Input: part model. Units: mm. Frame: model coordinates. Face numbers are marked on the shaded views. A direction names the side the tool comes from. Round coordinates to 2 decimals unless told otherwise and drop trailing zeros. Write each loop counter-clockwise with the first axis right and the second up, starting at its lowest first coordinate (ties: lowest second). Pieces come first, ordered by that corner, then holes. Notation, with made-up numbers: (61, 36.25) - (87, 36.25) arc R22 cw to (87, 74.25) - close; hole circle Ø5 at (78.25, 29). An arc over 180 degrees is marked (long way). Use one line per item in the form item = value.
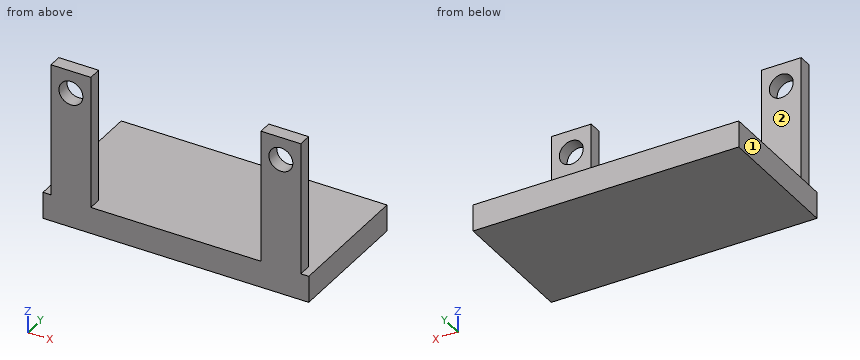
```python
from build123d import *

# Parameters (mm, degrees)
F1_DEPTH = 5.08
F0_W     = 7.62
F0_H     = 2.54
F2_DEPTH = 30.48
F3_R     = 2.286
F3_R_2   = 2.286002
F4_DEPTH = 7.112


with BuildPart() as f1:
    # F0 (on Top) → F1 (new body)
    with BuildSketch(Plane.XY):
        Polygon((25.4, 12.7), (-25.4, 12.7), (-25.4, -12.7), (-23.876, -12.7), (-23.876, -10.16), (-16.256, -10.16), (-16.256, -12.7), (16.256, -12.7), (16.256, -10.16), (23.876, -10.16), (23.876, -12.7), (25.4, -12.7), align=None)
    extrude(amount=F1_DEPTH)

    # F0 (on Top) → F2 (join)
    with BuildSketch(Plane.XY):
        with Locations((-20.066, -11.43)):
            Rectangle(F0_W, F0_H)
        with Locations((20.066, -11.43)):
            Rectangle(F0_W, F0_H)
    extrude(amount=F2_DEPTH)

    # F3 (on face) → F4 (cut)
    with BuildSketch(Plane(origin=(0, -10.16, 0), x_dir=(-1, 0, 0), z_dir=(0, 1, 0))):
        with Locations((-20.066, 26.162)):
            Circle(F3_R)
        with Locations((20.066, 26.162)):
            Circle(F3_R_2)
    extrude(amount=-F4_DEPTH, mode=Mode.SUBTRACT)


solid = f1.part
```
(1) Access query for the marked faces 1 and 2. Directions: +Z, -Z, +X, -X, +Y, -Y. A direction counts if a zero-diameter tool reaches every point of the face in a straight line with its end or side. Return the directions, or none.
Derived:
face_1 = +Z, -Z, -X, +Y, -Y
face_2 = +Z, +X, -X, +Y
(2) First-contact query: pin 1 Ø6 at (x, z) = (-20.066, 26.162) entering from +Y; pin 2 Ø2 at (y, z) = (-11.5, 12.5) entering from +X; pin 3 Ø1.5 at (x, y) = (-7.5, -3.5) entering from +Z. Flat tips, straight axial feed; report the tip coordinate or a pass-through.
Derived:
pin_1 = -10.16
pin_2 = 23.88
pin_3 = 5.08
(3) Cut plane B-B on y = -0.75. Output: boundary loops of the cut face in (x, z), then the cut area to 3 significant figures.
Derived:
outline = (-25.4, 0) - (25.4, 0) - (25.4, 5.08) - (-25.4, 5.08) - close
area = 258 mm^2
(4) Cut plane C-C on x = 5. Output: boundary loops of the cut face in (y, z), then the cut area to 3 significant figures.
Derived:
outline = (-12.7, 0) - (12.7, 0) - (12.7, 5.08) - (-12.7, 5.08) - close
area = 129 mm^2
(5) Material intervals for L1, parallel to X at y = -10.75, z = 15; L2, parallel to Z at x = -14, y = 8.5; L3, parallel to Y at x = -22, z = 17, sorted ascending.
Derived:
L1 = -23.88 to -16.26, 16.26 to 23.88
L2 = 0 to 5.08
L3 = -12.7 to -10.16
(6) Cut plane A-A on z = 29. Output: boundary loops of the cut face in (x, y).
Derived:
outline = (-23.88, -12.7) - (-16.26, -12.7) - (-16.26, -10.16) - (-23.88, -10.16) - close; (16.26, -12.7) - (23.88, -12.7) - (23.88, -10.16) - (16.26, -10.16) - close
